from build123d import *

# Parameters (mm, degrees)
F0_W     = 60.325
F0_H     = 9.525
F0_R     = 0.8509
F0_R_2   = 3.175
F1_DEPTH = 12.7
F3_DEPTH = 9.526


# Not quite as in the source:
# - a feature of the source that left no trace in its solid (it failed there, or was rolled back) is left out


with BuildPart() as f1:
    # F0 (on Front) → F1 (new body)
    with BuildSketch(Plane.XZ):
        with Locations((30.1625, 4.7625)):
            Rectangle(F0_W, F0_H)
        with Locations((3.175, 4.7625)):
            Circle(F0_R, mode=Mode.SUBTRACT)
        with Locations((53.975, 4.7625)):
            Circle(F0_R_2, mode=Mode.SUBTRACT)
    extrude(amount=-F1_DEPTH)

    # F2 (on face) → F3 (cut, through all)
    with BuildSketch(Plane.XY.offset(9.525)):
        with BuildLine():
            Line((10.99566, 8.33374), (0, 8.33374))
            Line((0, 8.33374), (0, 4.36626))
            Line((0, 4.36626), (10.99566, 4.36626))
            ThreePointArc((10.99566, 4.36626), (12.3983760061, 4.9472839939), (12.9794, 6.35))
            ThreePointArc((12.9794, 6.35), (12.3983760061, 7.7527160061), (10.99566, 8.33374))
        make_face()
    extrude(amount=-F3_DEPTH, mode=Mode.SUBTRACT)


solid = f1.part
Design review of the part built by this model. Coordinates are the model's own, in mm. A direction names the side the tool comes from. Coordinates: 2 decimals unless noted, no trailing zeros. Order: outer loops, then holes, each group sorted by start corner. A loop starts at its lowest first (then second) coordinate and runs counter-clockwise, first axis right, second up. Notation, with made-up numbers: (87.25, 51) -> (141.25, 51) arc R20 cw to (141.25, 58) -> close; hole circle Ø3 at (-37.75, -35). An arc over 180 degrees is marked (long way). One line per item, written item: value.
1) Draft analysis for pull direction X (two halves, no side actions). For faces 1 (the face through (30, 6, 0)), 2 (the face through (60.325, 6, 5)), 3 (the face through (3.6, 10.5, 5.5)), state which applies: +X half, -X half, draft (parallel to the pull), parting line (faces both ways), or undercut.
Output values:
face 1: draft
face 2: +X half
face 3: undercut
2) We need section A-A, the plane x = 7.5. Give the boundary of the cut face in (y, z) (3 decimals).
Output values:
outline: (0, 0) -> (4.366, 0) -> (4.366, 9.525) -> (0, 9.525) -> close; (8.334, 0) -> (12.7, 0) -> (12.7, 9.525) -> (8.334, 9.525) -> close
3) We need section D-D, the plane x = 55.5. Give the boundary of the cut face in (y, z) (3 decimals).
Output values:
outline: (0, 0) -> (12.7, 0) -> (12.7, 1.978) -> (0, 1.978) -> close; (0, 7.547) -> (12.7, 7.547) -> (12.7, 9.525) -> (0, 9.525) -> close
4) We need section C-C, the plane y = 2.75. Count the separate pieces of the cut face and the enclosed holes in it, then the cut area to 3 significant figures.
Output values:
separate pieces: 1
enclosed holes: 2
area: 541 mm2
5) Machinability: for faces 4 (the face through (0, 2, 5)), 5 (the face through (5, 4.366, 5)), which of the approach directions +Z, -Z, +X, -X, +Y, -Y give a long, thin tool a straight path to every point of the face, cutting with its end or side? Answer none if there is none.
Output values:
face 4: +Z, -Z, -X, +Y, -Y
face 5: +Z, -Z, -X
6) To check wall thickness, follow probe 1 along Y at (x, z) = (11, 3.5); probe 2 along X at (y, z) = (5, 3) (3 decimals); probe 3 along X at (y, z) = (4, 7.25) (3 decimals). State the ranges of each line that lie inside material, in increasing order. Write a range as [from, to].
Output values:
probe 1: y = [0, 4.37], [8.33, 12.7]
probe 2: x = [12.449, 51.334], [56.616, 60.325]
probe 3: x = [0, 52.002], [55.948, 60.325]
7) We need section B-B, the plane z = 6.5. Give the boundary of the cut face in (x, y) (3 decimals).
Output values:
outline: (0, 0) -> (51.318, 0) -> (51.318, 12.7) -> (0, 12.7) -> (0, 8.334) -> (10.996, 8.334) arc R1.984 cw to (10.996, 4.366) -> (0, 4.366) -> close; (56.632, 0) -> (60.325, 0) -> (60.325, 12.7) -> (56.632, 12.7) -> close
8) Clearance check with a flat-ended pin moving along its axis: P1, Ø5.5, axis at x = 53.98, z = 4.76, coming from the +Y side. State where the tip first meets the part, or that it passes through.
Output values:
P1: passes through
